from build123d import *

# Parameters (mm, degrees)
SKETCH_1_R                 = 1.6
EXTRUDE_1_DEPTH            = 3
HOLE_WIZARD_2_D            = 3.3
PATTERN_LINEAR_1_COUNT     = 7
PATTERN_LINEAR_1_PITCH     = 20
PATTERN_LINEAR_1_COL_COUNT = 7
PATTERN_LINEAR_1_COL_PITCH = 20


with BuildPart() as part:
    # 草图1 → 凸台-拉伸1 (new body)
    with BuildSketch(Plane.XY):
        with BuildLine():
            Line((-61, 8.5), (61, 8.5))
            ThreePointArc((61, 8.5), (63.121320344, 7.621320344), (64, 5.5))
            Line((64, 5.5), (64, 0))
            Line((64, 0), (82, 0))
            Line((82, 0), (82, 5.5))
            ThreePointArc((82, 5.5), (82.878679656, 7.621320344), (85, 8.5))
            Line((85, 8.5), (131, 8.5))
            ThreePointArc((131, 8.5), (133.121320344, 9.378679656), (134, 11.5))
            Line((134, 11.5), (134, 30))
            Line((134, 30), (116, 30))
            Line((116, 30), (116, 24.5))
            ThreePointArc((116, 24.5), (115.121320344, 22.378679656), (113, 21.5))
            Line((113, 21.5), (-113, 21.5))
            ThreePointArc((-113, 21.5), (-115.121320344, 22.378679656), (-116, 24.5))
            Line((-116, 24.5), (-116, 30))
            Line((-116, 30), (-134, 30))
            Line((-134, 30), (-134, 11.5))
            ThreePointArc((-134, 11.5), (-133.121320344, 9.378679656), (-131, 8.5))
            Line((-131, 8.5), (-85, 8.5))
            ThreePointArc((-85, 8.5), (-82.878679656, 7.621320344), (-82, 5.5))
            Line((-82, 5.5), (-82, 0))
            Line((-82, 0), (-64, 0))
            Line((-64, 0), (-64, 5.5))
            ThreePointArc((-64, 5.5), (-63.121320344, 7.621320344), (-61, 8.5))
        make_face()
        with Locations((-77.5, 4.5)):
            Circle(SKETCH_1_R, mode=Mode.SUBTRACT)
        with Locations((-68.5, 4.5)):
            Circle(SKETCH_1_R, mode=Mode.SUBTRACT)
        with Locations((120.5, 25.5)):
            Circle(SKETCH_1_R, mode=Mode.SUBTRACT)
        with Locations((129.5, 25.5)):
            Circle(SKETCH_1_R, mode=Mode.SUBTRACT)
        with Locations((68.5, 4.5)):
            Circle(SKETCH_1_R, mode=Mode.SUBTRACT)
        with Locations((77.5, 4.5)):
            Circle(SKETCH_1_R, mode=Mode.SUBTRACT)
        with Locations((-129.5, 25.5)):
            Circle(SKETCH_1_R, mode=Mode.SUBTRACT)
        with Locations((-120.5, 25.5)):
            Circle(SKETCH_1_R, mode=Mode.SUBTRACT)
    extrude(amount=EXTRUDE_1_DEPTH)

    # 孔2 (through all)
    with Locations(Plane(origin=(0, 0, 0), x_dir=(-1, 0, 0), z_dir=(0, 0, -1))):
        with Locations((0, 14.5)):
            hole_wizard_2 = Hole(HOLE_WIZARD_2_D / 2)

    # 阵列(线性)1: 孔2 ×7
    with Locations(*[(i * PATTERN_LINEAR_1_PITCH, 0, 0) for i in range(1, PATTERN_LINEAR_1_COUNT)]):
        add(hole_wizard_2, mode=Mode.SUBTRACT)

    # 阵列(线性)1 col: 孔2 ×7
    with Locations(*[(-i * PATTERN_LINEAR_1_COL_PITCH, 0, 0) for i in range(1, PATTERN_LINEAR_1_COL_COUNT)]):
        add(hole_wizard_2, mode=Mode.SUBTRACT)


solid = part.part
Geometry check sheet. Reference: the model listing, model coordinates, mm. Give positions to 0.01 mm unless a question says otherwise; leave off trailing zeros. Write each loop counter-clockwise with the first axis right and the second up, starting at its lowest first coordinate (ties: lowest second). Pieces come first, ordered by that corner, then holes. Notation, with made-up numbers: M 28.5,-30 L 65.5,-30 A24 cw 65.5,1 Z; hole C -29.75,-40 d9. An arc over 180 degrees is marked long. Answer as CSV lines item,"result". Start each with the question number.
Q1. Section check B-B, the plane x = 10.5. Record the cut outline in (y, z).
Q2. Section check A-A, the plane z = 0.55. Give the number of separate pieces and of enclosed holes in the cut face, then the cut area to 3 significant figures.
Q3. Material ranges on L1, parallel to X at y = 25.25, z = 1.1; L2, parallel to Y at x = 129.5, z = 1.2; L3, parallel to Y at x = -68.5, z = 0.7, recorded low to high.
Q4. Go/stop test with flat-tipped pins: pin 1 (2.5 mm diameter, centred on x = -77.5, y = 4.5, fed in from +Z); pin 2 (1.5 mm diameter, centred on x = -47, z = 0.5, fed in from -Y). Record where each tip stops, or that it passes through.
Geometry says:
1,outline,"M 8.5,0 L 21.5,0 L 21.5,3 L 8.5,3 Z"
2,separate pieces,"1"
2,enclosed holes,"21"
2,area,"3,930 mm^2"
3,L1,"-134 to -131.08, -127.92 to -122.08, -118.92 to -116, 116 to 118.92, 122.08 to 127.92, 131.08 to 134"
3,L2,"8.5 to 23.9, 27.1 to 30"
3,L3,"0 to 2.9, 6.1 to 21.5"
4,pin 1,"through"
4,pin 2,"y = 8.5"
